Part model, mm, in its own coordinate system. Face numbers are marked on the shaded views. A direction names the side the tool comes from. Give positions to 0.01 mm unless a question says otherwise; leave off trailing zeros. Order: outer loops, then holes, each group sorted by start corner. A loop starts at its lowest first (then second) coordinate and runs counter-clockwise, first axis right, second up. Notation, with made-up numbers: M 28,71.5 L 78,71.5 A17 ccw 78,89.5 Z; hole C -39.75,-21 d10. An arc over 180 degrees is marked long. One line per question, with ' | ' between items.
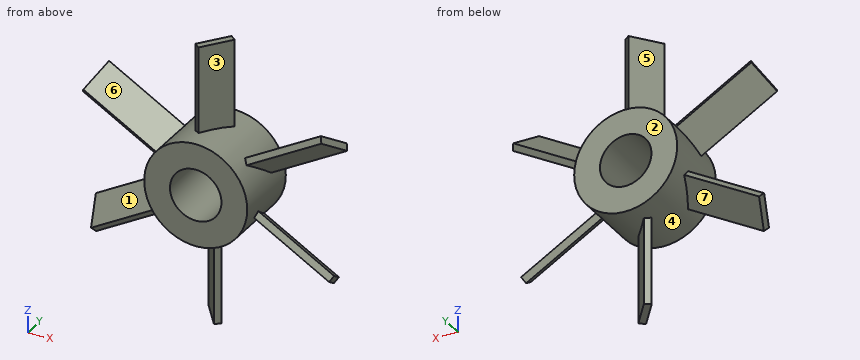
```python
from build123d import *

# Parameters (mm, degrees)
F1_DEPTH = 25.4
F3_COUNT = 6
F4_R     = 9.525
F5_DEPTH = 6.35
F6_R     = 4.7625
F7_DEPTH = 12.7


with BuildPart() as f1:
    # F0 (on Top) → F1 (new body)
    with BuildSketch(Plane.XY):
        Polygon((2.437655, 2.131124), (1.43048, 2.904751), (-2.437655, -2.131124), (-1.43048, -2.904751), align=None)
    extrude(amount=F1_DEPTH)



with BuildPart() as f3_1:
    # F3: instance of F1
    add(f1.part.rotate(Axis((0, 19.05, 0), (0, 1, 0)), 1 * 360 / F3_COUNT))


with BuildPart() as f3_2:
    # F3: instance of F1
    add(f1.part.rotate(Axis((0, 19.05, 0), (0, 1, 0)), 2 * 360 / F3_COUNT))


with BuildPart() as f3_3:
    # F3: instance of F1
    add(f1.part.rotate(Axis((0, 19.05, 0), (0, 1, 0)), 3 * 360 / F3_COUNT))


with BuildPart() as f3_4:
    # F3: instance of F1
    add(f1.part.rotate(Axis((0, 19.05, 0), (0, 1, 0)), 4 * 360 / F3_COUNT))


with BuildPart() as f3_5:
    # F3: instance of F1
    add(f1.part.rotate(Axis((0, 19.05, 0), (0, 1, 0)), 5 * 360 / F3_COUNT))


with BuildPart() as f1_1:
    add(f1.part)

    add(f3_1.part)  # F5 merges F3_1

    add(f3_2.part)  # F5 merges F3_2

    add(f3_3.part)  # F5 merges F3_3

    add(f3_4.part)  # F5 merges F3_4

    add(f3_5.part)  # F5 merges F3_5
    # F4 (on Front) → F5 (join, symmetric)
    with BuildSketch(Plane.XZ):
        Circle(F4_R)
    extrude(amount=F5_DEPTH, both=True)

    # F6 (on face) → F7 (cut)
    with BuildSketch(Plane.XZ.offset(6.35)):
        Circle(F6_R)
    extrude(amount=-F7_DEPTH, mode=Mode.SUBTRACT)


solid = f1_1.part
```
1. Mould opens along X. For the marked faces 1, 2 and 3 say: released by +X, released by -X, zero draft, split by the parting line, or undercut.
Worked out:
face 1: released by -X | face 2: zero draft | face 3: undercut
2. Slice it at B-B on x = -15.5. Give the cut face in (y, z), then the cut area to 3 significant figures.
Worked out:
outline: M -2.9,-10.6 L -2.13,-11.76 L 2.9,-7.3 L 2.13,-6.13 Z; M -2.9,7.3 L -2.13,6.13 L 2.9,10.6 L 2.13,11.76 Z | area: 18.6 mm2
3. Slice it at C-C on z = 22.5. Give the cut face in (x, y).
Worked out:
outline: M -2.44,-2.13 L -1.43,-2.9 L 2.44,2.13 L 1.43,2.9 Z
4. Probe L1, parallel to Z at x = 0, y = 1.75 (1 decimal); L2, parallel to Z at x = 0, y = 0.5; L3, parallel to X at y = -1.5, z = 11. List the from-to ranges inside material, lowest first. Write a range as from..to.
Worked out:
L1: z = -9.5..-4.8, 4.8..9.5 | L2: z = -25.4..-4.76, 4.76..25.4 | L3: x = -22.96..-19.76, -1.95..-0.35, 15.15..18.35
5. Tool access for the marked faces 4, 5, 6 and 7: list every direction of +Z, -Z, +X, -X, +Y, -Y with a clear straight run to the whole face (end or side of a thin tool).
Worked out:
face 4: none | face 5: +Z, +Y | face 6: +Z, -Y | face 7: -Z, +Y
6. Drop flat-ended pins along their axis: pin 1 (11 mm diameter, centred on x = 0, z = 0, fed in from +Y); pin 2 (2 mm diameter, centred on y = -2, z = 16, fed in from -X); pin 3 (4 mm diameter, centred on x = -4, z = -15, fed in from +Y); pin 4 (6 mm diameter, centred on y = 5, z = 11.5, fed in from -X). Give the stop position or say it passes through.
Worked out:
pin 1: stops at y = 6.35 | pin 2: stops at x = -2.44 | pin 3: stops at y = 2.47 | pin 4: stops at x = -20.78
